```python
from build123d import *

# Parameters (mm, degrees)
SKETCH1_W           = 86.32648043
SKETCH1_H           = 130
BOSS_EXTRUDE1_DEPTH = 5
CUT_EXTRUDE2_DEPTH  = 10
SKETCH4_R           = 1
CUT_EXTRUDE3_DEPTH  = 10


with BuildPart() as part:
    # Sketch1 → Boss-Extrude1 (new body)
    with BuildSketch(Plane.XY):
        with Locations((9.075669342, 37.952105326)):
            Rectangle(SKETCH1_W, SKETCH1_H)
    extrude(amount=BOSS_EXTRUDE1_DEPTH)

    # Sketch3 → Cut-Extrude2 (cut)
    with BuildSketch(Plane.XY.offset(5)):
        Polygon((-34.087570873, -18.047894674), (-27.087570873, -18.047894674), (-27.087570873, -17.297894674), (-24.687570873, -17.297894674), (-24.687570873, -18.047894674), (-17.087570873, -18.047894674), (-17.087570873, -22.047894674), (-24.687570873, -22.047894674), (-24.687570873, -22.797894674), (-27.087570873, -22.797894674), (-27.087570873, -22.047894674), (-34.087570873, -22.047894674), align=None)
        Polygon((52.238909557, -18.047894674), (52.238909557, -22.047894674), (45.238909557, -22.047894674), (45.238909557, -22.797894674), (42.838909557, -22.797894674), (42.838909557, -22.047894674), (35.238909557, -22.047894674), (35.238909557, -18.047894674), (42.838909557, -18.047894674), (42.838909557, -17.297894674), (45.238909557, -17.297894674), (45.238909557, -18.047894674), align=None)
        Polygon((52.238909557, 93.952105326), (45.238909557, 93.952105326), (45.238909557, 93.202105326), (42.838909557, 93.202105326), (42.838909557, 93.952105326), (35.238909557, 93.952105326), (35.238909557, 97.952105326), (42.838909557, 97.952105326), (42.838909557, 98.702105326), (45.238909557, 98.702105326), (45.238909557, 97.952105326), (52.238909557, 97.952105326), align=None)
        Polygon((-34.087570873, 93.952105326), (-34.087570873, 97.952105326), (-27.087570873, 97.952105326), (-27.087570873, 98.702105326), (-24.687570873, 98.702105326), (-24.687570873, 97.952105326), (-17.087570873, 97.952105326), (-17.087570873, 93.952105326), (-24.687570873, 93.952105326), (-24.687570873, 93.202105326), (-27.087570873, 93.202105326), (-27.087570873, 93.952105326), align=None)
    extrude(amount=-CUT_EXTRUDE2_DEPTH, mode=Mode.SUBTRACT)

    # Sketch4 → Cut-Extrude3 (cut)
    with BuildSketch(Plane.XY.offset(5)):
        with Locations((40.075669342, 1.232918464)):
            Circle(SKETCH4_R)
        with Locations((-21.924330658, 1.232918464)):
            Circle(SKETCH4_R)
        with Locations((-15.924330658, 58.232918464)):
            Circle(SKETCH4_R)
        with Locations((34.075669342, 58.232918464)):
            Circle(SKETCH4_R)
    extrude(amount=-CUT_EXTRUDE3_DEPTH, mode=Mode.SUBTRACT)


solid = part.part
```
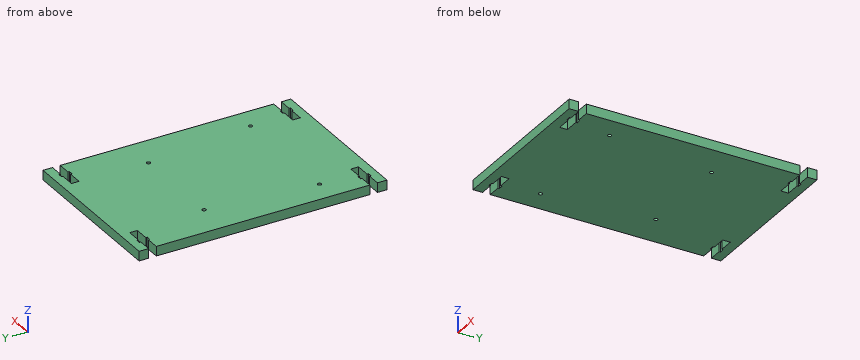
For this review, take the finished solid that the model builds, in its own axes (mm). Round coordinates to 2 decimals unless told otherwise and drop trailing zeros.
Q1. Insertion check: pin 1 Ø2.5 at (x, y) = (40.08, 1.23) entering from -Z. The pin has a flat end and moves straight along its axis. Give the tip position at first contact, or say it passes through.
Result sheet:
pin 1: stops at z = 0
Q2. Add section A-A on z = 3.3. Give the number of separate pieces and of enclosed holes in the cut face, plus the area to 3 significant figures.
Result sheet:
separate pieces: 1
enclosed holes: 4
area: 10,900 mm2
Q3. To check wall thickness, follow line 1 along Y through (x, z) = (-28, 3.4); line 2 along Y through (x, z) = (44.5, 2.45); line 3 along Y through (x, z) = (40, 2.5). State the ranges of each line that lie inside material, in increasing order.
Result sheet:
line 1: y = -27.05 to -22.05, -18.05 to 93.95, 97.95 to 102.95
line 2: y = -27.05 to -22.8, -17.3 to 93.2, 98.7 to 102.95
line 3: y = -27.05 to -22.05, -18.05 to 0.24, 2.23 to 93.95, 97.95 to 102.95
